Source: CAD feature listing. Evaluate the final solid. Frame: model axes, mm. A direction names the side the tool comes from. Give positions to 0.01 mm unless a question says otherwise; leave off trailing zeros. Write each loop counter-clockwise with the first axis right and the second up, starting at its lowest first coordinate (ties: lowest second). Pieces come first, ordered by that corner, then holes. Notation, with made-up numbers: (-8.5, 25.25) -> (48.5, 25.25) arc R17 ccw to (48.5, 30.25) -> close; hole circle Ø5 at (20, 22). An arc over 180 degrees is marked (long way). Answer as a JSON object with one key per item and string values. Group by question number.
Item 1: Access query for faces 1 (the face through (21, -3.048, 0)), 2 (the face through (-26.3, 0.64, 2.73)), 3 (the face through (-3.048, -21, 0)), 4 (the face through (21, 2.694, 0)), 5 (the face through (-17.906, 7.424, 13.501)). Directions: +Z, -Z, +X, -X, +Y, -Y. A direction counts if a zero-diameter tool reaches every point of the face in a straight line with its end or side. Return the directions, or none.
Item 2: First-contact query: pin 1 Ø1.5 at (x, z) = (-9, 28.5) entering from +Y; pin 2 Ø18.5 at (x, y) = (0, 2) entering from -Z; pin 3 Ø1.6 at (y, z) = (-21.5, 1.5) entering from -X. Flat tips, straight axial feed; report the tip coordinate or a pass-through.
Item 3: Ray query, probe 1 along Y at (x, z) = (0, 26.5); probe 2 along Y at (x, z) = (-1.5, 19). Return the intervals inside material, ascending. Write a range as from..to.
Item 4: Section query B-B on z = -5.5. Return the cut outline in (x, y), plus the area to 3 significant figures.
Item 5: Section query C-C on y = 27. Return the cut outline in (x, z).
Item 6: Pull-direction query (Y, two-part tool) for faces 6 (the face through (-10.902, -3.433, 14.212)), 7 (the face through (-7, 10, -11.543)), 8 (the face through (-0.64, -26.3, 2.73)); classes: pulls with the +Y half, pulls with the -Y half, needs draft (parallel to the pull), parting line crosses it, or undercut.
Item 7: Section query A-A on z = 37. Return the cut outline in (x, y), plus the area to 3 significant figures.
from build123d import *

# Parameters (mm, degrees)
F3_DEPTH = 23.622
F5_DEPTH = 267.208
F7_COUNT = 4


with BuildPart() as f1:
    # F0 (on Front) → F1 (revolve)
    with BuildSketch(Plane.XZ):
        Polygon((-11.43, -11.5434539532), (-11.43, 13.8565460468), (-11.43, 39.2565460468), (0, 39.2565460468), (0, 64.4025460468), (-19.3840445728, 39.2565460468), (-19.3840445728, -11.5434539532), align=None)
    revolve(axis=Axis((0, 0, 51.8295460468), (0, 0, 1)))

    # F2 (on face) → F3 (join)
    with BuildSketch(Plane(origin=(0, 0, -11.5434539532), x_dir=(1, 0, 0), z_dir=(0, 0, -1))):
        with BuildLine():
            Line((-2.6940780226, -19.1959143468), (-2.6940780226, -22.5224811584))
            Line((-2.6940780226, -22.5224811584), (0.1769623486, -33.5143171251))
            Line((0.1769623486, -33.5143171251), (3.0480027199, -22.3197587766))
            Line((3.0480027199, -22.3197587766), (3.0480027199, -19.1429063473))
            ThreePointArc((3.0480027199, -19.1429063473), (0.1789361194, -19.3832186663), (-2.6940780226, -19.1959143468))
        make_face()
    extrude(amount=-F3_DEPTH)

    # F4 (on face) → F5 (cut)
    with BuildSketch(Plane(origin=(-8.0291148796, 2.0971849502, 0), x_dir=(-0.2527189829, -0.9675397231, 0), z_dir=(-0.9675397231, 0.2527189829, 0))):
        Polygon((-32.4711548542, -11.5434539532), (-21.1105505247, 12.0785460468), (-32.4711548542, 12.0785460468), align=None)
    extrude(amount=-F5_DEPTH, mode=Mode.SUBTRACT)

    # F7: F1 ×4 about axis
    f7_axis = Axis((0, 0, 24.6183145791), (0, 0, -1))


with BuildPart() as f1_1:
    add(f1.part)
    for i in range(1, F7_COUNT):
        add(f1.part.rotate(f7_axis, i * 360 / F7_COUNT))


solid = f1_1.part
Worked answers:
{
 "1": {"face 1": "+Z, -Z, +X, -Y", "face 2": "+Z, -X, +Y", "face 3": "+Z, -Z, -X, -Y", "face 4": "+Z, -Z, +X, +Y", "face 5": "+Z"},
 "2": {"pin 1": "y = 17.54", "pin 2": "z = 39.26", "pin 3": "x = -3.05"},
 "3": {"probe 1": "-19.38..-11.43, 11.43..19.38", "probe 2": "-19.33..-11.33, 11.33..19.33"},
 "4": {"outline": "(-30.7, -0.56) -> (-22.52, -2.69) -> (-19.2, -2.69) arc R19.38 ccw to (-3.05, -19.14) -> (-3.05, -22.32) -> (-1, -30.29) -> (0.56, -30.7) -> (2.69, -22.52) -> (2.69, -19.2) arc R19.38 ccw to (19.14, -3.05) -> (22.32, -3.05) -> (30.29, -1) -> (30.7, 0.56) -> (22.52, 2.69) -> (19.2, 2.69) arc R19.38 ccw to (3.05, 19.14) -> (3.05, 22.32) -> (1, 30.29) -> (-0.56, 30.7) -> (-2.69, 22.52) -> (-2.69, 19.2) arc R19.38 ccw to (-19.14, 3.05) -> (-22.32, 3.05) -> (-30.29, 1) -> close; hole circle Ø22.86 at (0, 0)", "area": "959 mm^2"},
 "5": {"outline": "(-1.52, -11.54) -> (1.85, -11.54) -> (1.85, 0.68) -> (-1.52, 2.46) -> close"},
 "6": {"face 6": "undercut", "face 7": "needs draft", "face 8": "pulls with the -Y half"},
 "7": {"outline": "circle Ø38.77 at (0, 0); hole circle Ø22.86 at (0, 0)", "area": "770 mm^2"}
}
